The listing builds one solid part. Answer for the finished solid, in the listing's coordinates (mm). A direction names the side the tool comes from. Coordinates: 2 decimals unless noted, no trailing zeros. Write each loop counter-clockwise with the first axis right and the second up, starting at its lowest first coordinate (ties: lowest second). Pieces come first, ordered by that corner, then holes.
from build123d import *

# Parameters (mm, degrees)
SKETCH2_R           = 5
SKETCH2_R_2         = 10
BOSS_EXTRUDE2_DEPTH = 12
SKETCH3_R           = 5
BOSS_EXTRUDE3_DEPTH = 12
SKETCH4_R           = 10
BOSS_EXTRUDE4_DEPTH = 48
BOSS_EXTRUDE5_DEPTH = 12
SKETCH6_R           = 4.4
CUT_EXTRUDE1_DEPTH  = 100.572444927


with BuildPart() as part:
    # Sketch2 → Boss-Extrude2 (new body)
    with BuildSketch(Plane.XY):
        with BuildLine():
            Line((0, 0), (-50, 0))
            Line((-50, 0), (-50, 90))
            ThreePointArc((-50, 90), (-47.071067812, 97.071067812), (-40, 100))
            Line((-40, 100), (-8, 100))
            Line((-8, 100), (-8, 96.572444927))
            Line((-8, 96.572444927), (8, 96.572444927))
            Line((8, 96.572444927), (8, 99.572444927))
            Line((8, 99.572444927), (60, 99.572444927))
            Line((60, 99.572444927), (60, 84.572444927))
            Line((60, 84.572444927), (48, 84.572444927))
            Line((48, 84.572444927), (48, 72.572444927))
            ThreePointArc((48, 72.572444927), (21.800398408, 50.444890038), (12, 17.581536588))
            Line((12, 17.581536588), (12, 0))
            Line((12, 0), (0, 0))
        make_face()
        with Locations((-40, 90)):
            Circle(SKETCH2_R, mode=Mode.SUBTRACT)
        with Locations((0, 80)):
            Circle(SKETCH2_R_2, mode=Mode.SUBTRACT)
    extrude(amount=BOSS_EXTRUDE2_DEPTH)

    # Sketch3 → Boss-Extrude3 (add)
    with BuildSketch(Plane.XZ):
        with BuildLine():
            Line((-50, 0), (-50, 38))
            ThreePointArc((-50, 38), (-47.071067812, 45.071067812), (-40, 48))
            Line((-40, 48), (12, 48))
            Line((12, 48), (12, 0))
            Line((12, 0), (-50, 0))
        make_face()
        with Locations((-40, 38)):
            Circle(SKETCH3_R, mode=Mode.SUBTRACT)
    extrude(amount=-BOSS_EXTRUDE3_DEPTH)

    # Sketch4 → Boss-Extrude4 (add)
    with BuildSketch(Plane.XY.offset(12)):
        with BuildLine():
            ThreePointArc((-15, 100), (-0.349804116, 55.002447378), (15.553758374, 99.572444927))
            Line((15.553758374, 99.572444927), (8, 99.572444927))
            Line((8, 99.572444927), (8, 96.572444927))
            Line((8, 96.572444927), (-8, 96.572444927))
            Line((-8, 96.572444927), (-8, 100))
            Line((-8, 100), (-15, 100))
        make_face()
        with Locations((0, 80)):
            Circle(SKETCH4_R, mode=Mode.SUBTRACT)
    extrude(amount=BOSS_EXTRUDE4_DEPTH)

    # Sketch5 → Boss-Extrude5 (add)
    with BuildSketch(Plane(origin=(0, 99.572444927, 0), x_dir=(1, 0, 0), z_dir=(0, 1, 0))):
        with BuildLine():
            Line((8, -60), (8, 0))
            Line((8, 0), (60, 0))
            Line((60, 0), (60, -12))
            Line((60, -12), (60, -30))
            ThreePointArc((60, -30), (51.213203436, -51.213203436), (30, -60))
            Line((30, -60), (8, -60))
        make_face()
    extrude(amount=-BOSS_EXTRUDE5_DEPTH)

    # Sketch6 → Cut-Extrude1 (cut, through all)
    with BuildSketch(Plane(origin=(0, 99.572444927, 0), x_dir=(1, 0, 0), z_dir=(0, 1, 0))):
        with Locations((31.202070331, -25.224562722)):
            Circle(SKETCH6_R)
    extrude(amount=-CUT_EXTRUDE1_DEPTH, mode=Mode.SUBTRACT)


solid = part.part
Q1. The part is cut by section C-C, the plane y = 80. Write down the section's boundary in (x, z).
Answers below:
outline: (-50, 0) - (-10, 0) - (-10, 60) - (-25, 60) - (-25, 12) - (-50, 12) - close; (10, 0) - (48, 0) - (48, 12) - (25, 12) - (25, 60) - (10, 60) - close
Q2. The part is cut by section A-A, the plane x = 0. Write down the section's boundary in (y, z), then the cut area to 3 significant figures.
Answers below:
outline: (0, 0) - (70, 0) - (70, 60) - (55, 60) - (55, 12) - (12, 12) - (12, 48) - (0, 48) - close; (90, 0) - (96.57, 0) - (96.57, 60) - (90, 60) - close
area: 2,390 mm2
Q3. Which of the six approach directions +Z, -Z, +X, -X, +Y, -Y give full straight-line access (tool end or side, diameter ignored) to faces 1 (the face through (-19, 12, 30)), 2 (the face through (-14, 6, 48)), 3 (the face through (-8, 98, 30)), 4 (the face through (12, 7, 24))?
Answers below:
face 1: +Z, +X, -X
face 2: +Z, +X, -X, -Y
face 3: +Z, -Z, +Y
face 4: +Z, -Z, +X, -Y
Q4. Find the intervals of material crossed by probe 1 along Y at (x, z) = (0, 34); probe 2 along Y at (x, z) = (-40, 6); probe 3 along Z at (x, y) = (-19, 49), in increasing order.
Answers below:
probe 1: y = 0 to 12, 55 to 70, 90 to 96.57
probe 2: y = 0 to 85, 95 to 100
probe 3: z = 0 to 12
Q5. Determine the mould class of faces 5 (the face through (8, 98, 30)), 6 (the face through (42, 87.572, 36)), 7 (the face through (-44, 87, 6)), 8 (the face through (-47.15, 5.92, 44.99)) for opening direction X: released by +X, released by -X, zero draft, split by the parting line, or undercut.
Answers below:
face 5: undercut
face 6: zero draft
face 7: undercut
face 8: released by -X
Q6. The part is cut by section B-B, the plane z = 16.5. Write down the section's boundary in (x, y).
Answers below:
outline: (-50, 0) - (12, 0) - (12, 12) - (-50, 12) - close; (-15, 100) arc R25 ccw (long way) to (23.83, 87.57) - (60, 87.57) - (60, 99.57) - (8, 99.57) - (8, 96.57) - (-8, 96.57) - (-8, 100) - close; hole circle Ø20 at (0, 80)
Q7. Given pin 1 (17.5 mm diameter, centred on x = -0.5, z = 24, fed in from +Y); pin 2 (13 mm diameter, centred on x = 56.5, z = 4.5, fed in from -Y); pin 3 (11 mm diameter, centred on x = 49, z = 28, fed in from -Y); pin 4 (1.5 mm diameter, centred on y = 98.5, z = 29.5, fed in from -X), each flat-ended and moving along its own axis, determine where each tip first touches the part or whether it passes through.
Answers below:
pin 1: stops at y = 100
pin 2: stops at y = 84.57
pin 3: stops at y = 87.57
pin 4: stops at x = -17.61
Q8. The part is cut by section D-D, the plane y = 93.5. Write down the section's boundary in (x, z).
Answers below:
outline: (-49.37, 0) - (-43.57, 0) - (-43.57, 12) - (-49.37, 12) - close; (-36.43, 0) - (60, 0) - (60, 30) arc R30 ccw to (30, 60) - (-21.04, 60) - (-21.04, 12) - (-36.43, 12) - close; hole circle Ø8.8 at (31.2, 25.22)
